from build123d import *

# Parameters (mm, degrees)
SKETCH1_R           = 1.5
BOSS_EXTRUDE1_DEPTH = 3
BOSS_EXTRUDE2_START = 22.5
SKETCH2_W           = 3.5
SKETCH2_H           = 6
BOSS_EXTRUDE2_DEPTH = 29
CHAMFER2_SIZE       = 2
SKETCH3_W           = 24
SKETCH3_H           = 29
SKETCH3_R           = 11
BOSS_EXTRUDE4_DEPTH = 7
CHAMFER3_SIZE       = 2


# Read off the part's stored shape, not the designer's step: Mirror1
with BuildPart() as part:
    # Sketch1 → Boss-Extrude1 (new body)
    with BuildSketch(Plane(origin=(0, 0, 0), x_dir=(1, 0, 0), z_dir=(0, 1, 0))):
        Polygon((-6, 17), (-3, 20), (3, 20), (6, 17), (6, -17), (3, -20), (-3, -20), (-6, -17), align=None)
        with Locations(Location((0, 14, 0), (0, 0, 270))):
            Circle(SKETCH1_R, mode=Mode.SUBTRACT)
        with Locations(Location((0, -14, 0), (0, 0, 270))):
            Circle(SKETCH1_R, mode=Mode.SUBTRACT)
    extrude(amount=BOSS_EXTRUDE1_DEPTH)

    # Sketch2 → Boss-Extrude2 (add)
    with BuildSketch(Plane(origin=(0, 3, 0), x_dir=(1, 0, 0), z_dir=(0, 1, 0)).offset(BOSS_EXTRUDE2_START)):
        with Locations((-7.75, 9)):
            Rectangle(SKETCH2_W, SKETCH2_H)
        with Locations((-7.75, -9)):
            Rectangle(SKETCH2_W, SKETCH2_H)
    extrude(amount=-BOSS_EXTRUDE2_DEPTH)

    # Chamfer2
    chamfer2_edges = [part.edges().sort_by_distance(p)[0] for p in [
        (-6, 0, -9),
        (-6, 0, 9),
        (-6, 3, -9),
        (-6, 3, 9),
    ]]
    chamfer(chamfer2_edges, length=CHAMFER2_SIZE)

    # Sketch3 → Boss-Extrude4 (add)
    with BuildSketch(Plane.ZY.offset(9.5)):
        with Locations((0, 11)):
            Rectangle(SKETCH3_W, SKETCH3_H)
        with Locations(Location((0, 11, 0), (0, 0, 236.944268849))):
            Circle(SKETCH3_R, mode=Mode.SUBTRACT)
    extrude(amount=BOSS_EXTRUDE4_DEPTH)

    # Chamfer3
    chamfer3_edges = [part.edges().sort_by_distance(p)[0] for p in [
        (-11.25, 25.5, -12),
        (-11.25, -3.5, -12),
        (-11.25, -3.5, 12),
        (-11.25, 25.5, 12),
    ]]
    chamfer(chamfer3_edges, length=CHAMFER3_SIZE)

    # Mirror1: part across plane


with BuildPart() as part_1:
    add(part.part)
    add(part.part.mirror(Plane(origin=(0, 11, 0), x_dir=(0, 0, 1), z_dir=(0, -1, 0))))


solid = part_1.part
Read the model definition and answer for the solid it produces. Units are mm, in the model's axes. A direction names the side the tool comes from. Give positions to 0.01 mm unless a question says otherwise; leave off trailing zeros. Write each loop counter-clockwise with the first axis right and the second up, starting at its lowest first coordinate (ties: lowest second). Pieces come first, ordered by that corner, then holes. Notation, with made-up numbers: (10.25, -5.5) - (69.25, -5.5) arc R7 cw to (69.25, 5.5) - close; hole circle Ø1 at (-20, 58.25). An arc over 180 degrees is marked (long way). Answer in a Markdown table with one row per item. Add a question column.
Item 1: Find the intervals of material crossed by L1, parallel to X at y = 20, z = -14; L2, parallel to Y at x = 2.25, z = 9; L3, parallel to Z at x = -12, y = 11, in increasing order.
Item 2: A tool of negligible diameter and unlimited length cuts with its end or side. For faces 4 (the face through (-9.5, 23, 0)), 5 (the face through (-12.951, 0.404, -2.954)), 6 (the face through (-6, -3, 8)), 7 (the face through (-6, 21, 15)), 8 (the face through (-6, 1, -14)), from which of +Z, -Z, +X, -X, +Y, -Y can it reach the whole face along a straight path? Write none if from no direction.
Item 3: Section C-C, the plane z = -14 is taken. Write down the section's boundary in (x, y), and give its area (3 significant figures).
Item 4: Section A-A, the plane y = 11 is taken. Write down the section's boundary in (x, z), and give its area (3 significant figures).
Item 5: Flat-ended cylindrical pins translate along their axes: P1, Ø4, axis at y = 15, z = -15.5, coming from the -X side; P2, Ø4, axis at x = -0.5, z = 15.5, coming from the -Y side; P3, Ø3.5, axis at x = 0, z = -14, coming from the +Y side; P4, Ø1.5, axis at y = 11, z = -9, coming from the -X side. Find the tip coordinate at first contact, or state that the pin passes through.
Item 6: Section B-B, the plane x = -8 is taken. Write down the section's boundary in (y, z).
Item 7: Determine the mould class of faces 1 (the face through (0, 0, 0)), 2 (the face through (0, 21, -20)), 3 (the face through (-5, 18, -9)) for opening direction Y: pulls with the +Y half, pulls with the -Y half, needs draft (parallel to the pull), parting line crosses it, or undercut.
Item 8: Section D-D, the plane x = 0 is taken. Write down the section's boundary in (y, z), and give its area (3 significant figures).
Recorded:
| question | item | result |
|---|---|---|
| 1 | L1 | x = -6 to -1.5, 1.5 to 6 |
| 1 | L2 | y = 0 to 3, 19 to 22 |
| 1 | L3 | z = -12 to -11, 11 to 12 |
| 2 | face 4 | +Y, -Y |
| 2 | face 5 | -X |
| 2 | face 6 | +Z, -Z, +X, -Y |
| 2 | face 7 | +Z, -X, +Y, -Y |
| 2 | face 8 | -Z, -X, +Y, -Y |
| 3 | outline | (-6, 0) - (-1.5, 0) - (-1.5, 3) - (-6, 3) - close; (-6, 19) - (-1.5, 19) - (-1.5, 22) - (-6, 22) - close; (1.5, 0) - (6, 0) - (6, 3) - (1.5, 3) - close; (1.5, 19) - (6, 19) - (6, 22) - (1.5, 22) - close |
| 3 | area | 54.0 mm2 |
| 4 | outline | (-16.5, -12) - (-6, -12) - (-6, -6) - (-9.5, -6) - (-9.5, -11) - (-16.5, -11) - close; (-16.5, 11) - (-9.5, 11) - (-9.5, 6) - (-6, 6) - (-6, 12) - (-16.5, 12) - close |
| 4 | area | 56.0 mm2 |
| 5 | P1 | passes through |
| 5 | P2 | stops at y = 0 |
| 5 | P3 | stops at y = 22 |
| 5 | P4 | stops at x = -9.5 |
| 6 | outline | (-3.5, -10) - (-1.5, -12) - (23.5, -12) - (25.5, -10) - (25.5, -6) - (-3.5, -6) - close; (-3.5, 6) - (25.5, 6) - (25.5, 10) - (23.5, 12) - (-1.5, 12) - (-3.5, 10) - close |
| 7 | face 1 | pulls with the -Y half |
| 7 | face 2 | needs draft |
| 7 | face 3 | undercut |
| 8 | outline | (0, -20) - (3, -20) - (3, -15.5) - (0, -15.5) - close; (0, -12.5) - (3, -12.5) - (3, 12.5) - (0, 12.5) - close; (0, 15.5) - (3, 15.5) - (3, 20) - (0, 20) - close; (19, -20) - (22, -20) - (22, -15.5) - (19, -15.5) - close; (19, -12.5) - (22, -12.5) - (22, 12.5) - (19, 12.5) - close; (19, 15.5) - (22, 15.5) - (22, 20) - (19, 20) - close |
| 8 | area | 204 mm2 |
